For this review, take the finished solid that the model builds, in its own axes (mm). A direction names the side the tool comes from. Coordinates: 2 decimals unless noted, no trailing zeros. Write each loop counter-clockwise with the first axis right and the second up, starting at its lowest first coordinate (ties: lowest second). Pieces come first, ordered by that corner, then holes. Notation, with made-up numbers: (34.25, 37.25) -> (46.25, 37.25) arc R27 cw to (46.25, 76.25) -> close; hole circle Ø10 at (79.5, 18.25). An arc over 180 degrees is marked (long way). One line per item, written item: value. Start each with the question number.
1) Add section B-B (z = 0). State the section outline as (x, y) points (1 decimal), and give its area (3 significant figures).
2) For pin 1 Ø1 at (x, z) = (15.5, -3) entering from +Y; pin 2 Ø3 at (x, y) = (-9, 3) entering from -Z; pin 3 Ø1 at (x, z) = (-11, -16.5) entering from +Y, all flat-tipped, find the tip position at first contact; note any pin that passes through.
3) Mouldability with a two-part tool opening along X and no side actions: class faces 4 (the flat face through (-28.575, 5, 0)), 5 (the cylindrical face through (-15.766, -24.796, 5.506)), 6 (the conical face through (28.34, 6.22, -19.76)), 7 (the cylindrical face through (-0.044, -5.796, 7.559)) as released by +X, released by -X, zero draft, split by the parting line, or undercut.
4) Add section C-C (x = -24.5). State the section outline as (y, z) points (1 decimal).
5) For probe 1 along X at (y, z) = (-14, 13) (3 decimals); probe 2 along X at (y, z) = (-3, 20.5); probe 3 along Y at (x, z) = (-1, -1), list the stretches that pass through material, from the lowest coordinate up. Write a range as from..to.
6) Add section A-A (x = -13). State the section outline as (y, z) points, and give its area (3 significant figures).
7) Machinability: for faces 1 (the conical face through (-28.34, 6.22, -19.76)), 2 (the flat face through (3.175, -4, -9)), 3 (the flat face through (0.4, -2.41, -4.11)), which of the approach directions +Z, -Z, +X, -X, +Y, -Y give a long, thin tool a straight path to every point of the face, cutting with its end or side? Answer none if there is none.
from build123d import *

# Parameters (mm, degrees)
BOSS_EXTRUDE1_START = -3.175
SKETCH1_R           = 25.4
BOSS_EXTRUDE1_DEPTH = 25.4
BOSS_EXTRUDE3_START = 3.175
SKETCH1_3_R         = 25.4
BOSS_EXTRUDE3_DEPTH = 25.4
CHAMFER1_SIZE       = 4.92
CHAMFER2_SIZE       = 4.92
SKETCH2_R           = 9.525
BOSS_EXTRUDE4_DEPTH = 6.35
CUT_EXTRUDE1_DEPTH  = 58.15


with BuildPart() as part:
    # Sketch1 → Boss-Extrude1 (new body)
    with BuildSketch(Plane(origin=(0, 0, 0), x_dir=(0, 0, -1), z_dir=(1, 0, 0)).offset(BOSS_EXTRUDE1_START)):
        Circle(SKETCH1_R)
    extrude(amount=-BOSS_EXTRUDE1_DEPTH)

    # Chamfer1
    chamfer1_edges = [part.edges().sort_by_distance(p)[0] for p in [
        (-3.175, 0, 25.4),
        (-28.575, 0, 25.4),
    ]]
    chamfer(chamfer1_edges, length=CHAMFER1_SIZE)



with BuildPart() as body_2:
    # Sketch1<3> → Boss-Extrude3 (new body)
    with BuildSketch(Plane(origin=(0, 0, 0), x_dir=(0, 0, -1), z_dir=(1, 0, 0)).offset(BOSS_EXTRUDE3_START)):
        Circle(SKETCH1_3_R)
    extrude(amount=BOSS_EXTRUDE3_DEPTH)

    # Chamfer2
    chamfer2_edges = [body_2.edges().sort_by_distance(p)[0] for p in [
        (3.175, 0, 25.4),
        (28.575, 0, 25.4),
    ]]
    chamfer(chamfer2_edges, length=CHAMFER2_SIZE)


with BuildPart() as part_1:
    add(part.part)

    add(body_2.part)  # Boss-Extrude4 merges body 2
    # Sketch2 → Boss-Extrude4 (add)
    with BuildSketch(Plane(origin=(-3.175, 0, 0), x_dir=(0, 0, -1), z_dir=(1, 0, 0))):
        Circle(SKETCH2_R)
    extrude(amount=BOSS_EXTRUDE4_DEPTH)

    # Sketch3 → Cut-Extrude1 (cut, through all)
    with BuildSketch(Plane(origin=(28.575, 0, 0), x_dir=(0, 0, -1), z_dir=(1, 0, 0))):
        Polygon((2.749630657, -4.7625), (5.499261314, 0), (2.749630657, 4.7625), (-2.749630657, 4.7625), (-5.499261314, 0), (-2.749630657, -4.7625), align=None)
    extrude(amount=-CUT_EXTRUDE1_DEPTH, mode=Mode.SUBTRACT)


solid = part_1.part
Numbers:
1. outline: (-28.6, -20.5) -> (-23.7, -25.4) -> (-8.1, -25.4) -> (-3.2, -20.5) -> (-3.2, -9.5) -> (3.2, -9.5) -> (3.2, -20.5) -> (8.1, -25.4) -> (23.7, -25.4) -> (28.6, -20.5) -> (28.6, -4.8) -> (-28.6, -4.8) -> close; (-28.6, 4.8) -> (28.6, 4.8) -> (28.6, 20.5) -> (23.7, 25.4) -> (8.1, 25.4) -> (3.2, 20.5) -> (3.2, 9.5) -> (-3.2, 9.5) -> (-3.2, 20.5) -> (-8.1, 25.4) -> (-23.7, 25.4) -> (-28.6, 20.5) -> close
1. area: 2,060 mm²
2. pin 1: y = 25.28
2. pin 2: z = -25.36
2. pin 3: y = 19.73
3. face 4: released by -X
3. face 5: zero draft
3. face 6: released by +X
3. face 7: undercut
4. outline: circle Ø49.1 at (0, 0); hole (-4.8, -2.7) -> (0, -5.5) -> (4.8, -2.7) -> (4.8, 2.7) -> (0, 5.5) -> (-4.8, 2.7) -> close
5. probe 1: -28.575..-3.175, 3.175..28.575
5. probe 2: -28.34..-3.41, 3.41..28.34
5. probe 3: -9.47..-4.76, 4.76..9.47
6. outline: circle Ø50.8 at (0, 0); hole (-4.76, -2.75) -> (0, -5.5) -> (4.76, -2.75) -> (4.76, 2.75) -> (0, 5.5) -> (-4.76, 2.75) -> close
6. area: 1,950 mm²
7. face 1: -X
7. face 2: none
7. face 3: +X, -X
